Here's the drawing with two shaded views (mm, measured from the low corner). I have some questions. Round coordinates to 2 decimals unless told otherwise and drop trailing zeros. Write each loop counter-clockwise with the first axis right and the second up, starting at its lowest first coordinate (ties: lowest second). Pieces come first, ordered by that corner, then holes. Notation, with made-up numbers: (49, 50) -> (87, 50) arc R13 cw to (87, 72) -> close; hole circle Ø7 at (-33, -35). An arc over 180 degrees is marked (long way). Use CSV: the item, a comma, the result in double quotes.
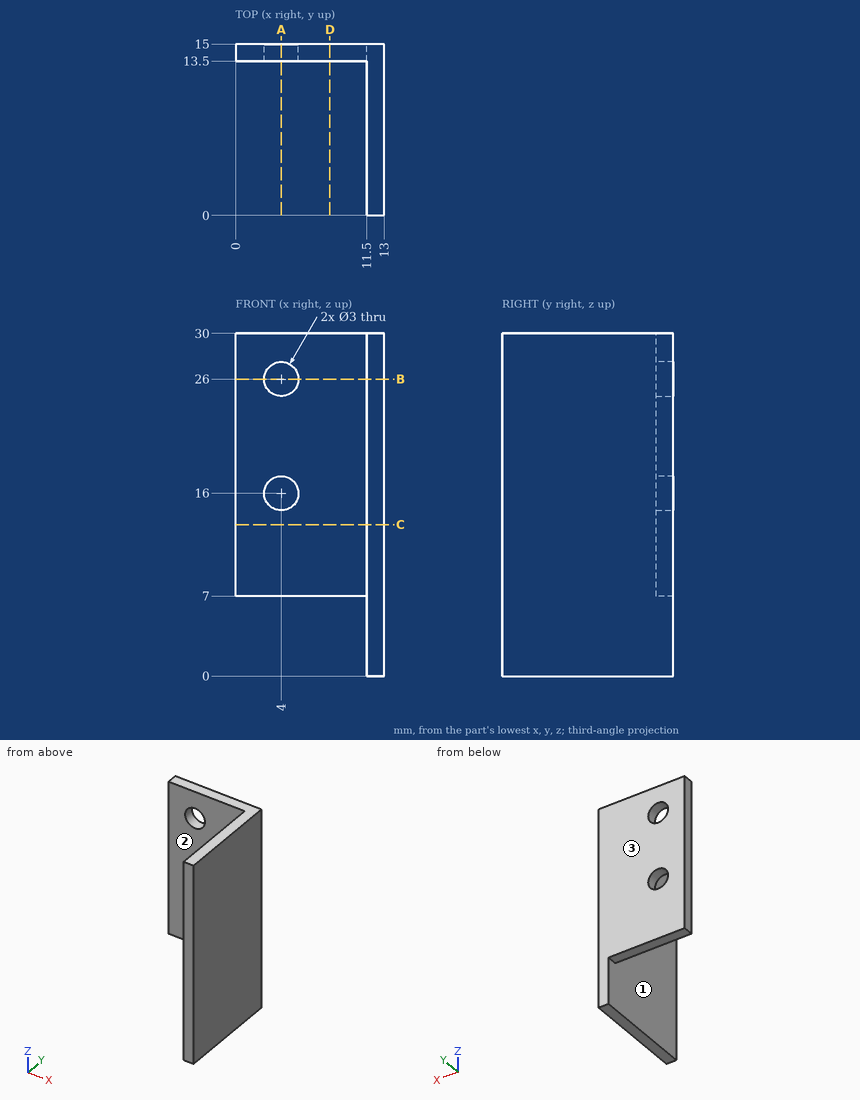
Q1. Suppose I cut it at C-C (z = 13.25). Write out the boundary of the cut face in (x, y), and give its area (4 significant figures).
Resolved:
outline,"(0, 13.5) -> (11.5, 13.5) -> (11.5, 0) -> (13, 0) -> (13, 15) -> (0, 15) -> close"
area,"39.75 mm^2"
Q2. Suppose I cut it at D-D (x = 8.25). Write out the boundary of the cut face in (y, z).
Resolved:
outline,"(13.5, 7) -> (15, 7) -> (15, 30) -> (13.5, 30) -> close"
Q3. Suppose I cut it at A-A (x = 4). Write out the boundary of the cut face in (y, z).
Resolved:
outline,"(13.5, 7) -> (15, 7) -> (15, 14.5) -> (13.5, 14.5) -> close; (13.5, 17.5) -> (15, 17.5) -> (15, 24.5) -> (13.5, 24.5) -> close; (13.5, 27.5) -> (15, 27.5) -> (15, 30) -> (13.5, 30) -> close"
Q4. Will these pins go through, and if not, where does the flat tip stop? P1, Ø3.5, axis at x = 4, z = 26, coming from the -Y side; P2, Ø4.5, axis at y = 5.5, z = 11.5, coming from the -X side.
Resolved:
P1,"stops at y = 13.5"
P2,"stops at x = 11.5"
Q5. Suppose I cut it at B-B (z = 26). Write out the boundary of the cut face in (x, y), and give its area (4 significant figures).
Resolved:
outline,"(0, 13.5) -> (2.5, 13.5) -> (2.5, 15) -> (0, 15) -> close; (5.5, 13.5) -> (11.5, 13.5) -> (11.5, 0) -> (13, 0) -> (13, 15) -> (5.5, 15) -> close"
area,"35.25 mm^2"
Q6. Please list where these lines run through material, in increasing order: probe 1 along Z at (x, y) = (4, 13.8); probe 2 along X at (y, z) = (13.9, 16); probe 3 along Y at (x, z) = (6, 18.25).
Resolved:
probe 1,"z = 7 to 14.5, 17.5 to 24.5, 27.5 to 30"
probe 2,"x = 0 to 2.5, 5.5 to 13"
probe 3,"y = 13.5 to 15"
Q7. If we mould it in two halves opening along Y, with no side actions, what happens to the marked faces 1, 2 and 3? For each: released by +Y, released by -Y, zero draft, split by the parting line, or undercut.
Resolved:
face 1,"zero draft"
face 2,"released by -Y"
face 3,"released by +Y"
